Drawing for the job (mm, zero at the part's lowest x, y, z). A direction names the side the tool comes from. Coordinates: 2 decimals unless noted, no trailing zeros. Order: outer loops, then holes, each group sorted by start corner. A loop starts at its lowest first (then second) coordinate and runs counter-clockwise, first axis right, second up. Notation, with made-up numbers: M 81.25,-33.75 L 117.25,-33.75 A29 cw 117.25,-13.75 Z; hole C 7.25,-16 d7. An arc over 180 degrees is marked long. Write item = value, one per line. Start each with the question number.
Q1. Pull direction Z, two halves, no side cores. Call the marked faces 1, 2 and 3: released by +Z, released by -Z, zero draft, split by the parting line, or undercut.
Q2. 3-axis set-ups, long thin cutter, end or side, ignore diameter. For the marked faces 4 and 5: which of +Z, -Z, +X, -X, +Y, -Y reach the whole face in a straight line?
Q3. Band-saw the part on C-C on x = 7.5. Write the cut outline in (y, z).
Q4. Band-saw the part on B-B on x = 32. Write the cut outline in (y, z).
Q5. Drill centre lines: probe 1 along Z at (x, y) = (3, 13.5) (1 decimal); probe 2 along Z at (x, y) = (23.5, 14.5) (1 decimal); probe 3 along Z at (x, y) = (19.5, 15.75). Where is each one in solid material? Low to high.
Q6. Band-saw the part on A-A on x = 3.5. Write the cut outline in (y, z) (1 decimal).
Q7. Pin check, flat tips, straight feed: P1, Ø6, axis at y = 24.5, z = 15.5, coming from the +X side (1 decimal); P2, Ø3, axis at x = 3, z = 13, coming from the -Y side; P3, Ø4, axis at x = 25.5, z = 9, coming from the +Y side. Stop position of each tip, or through.
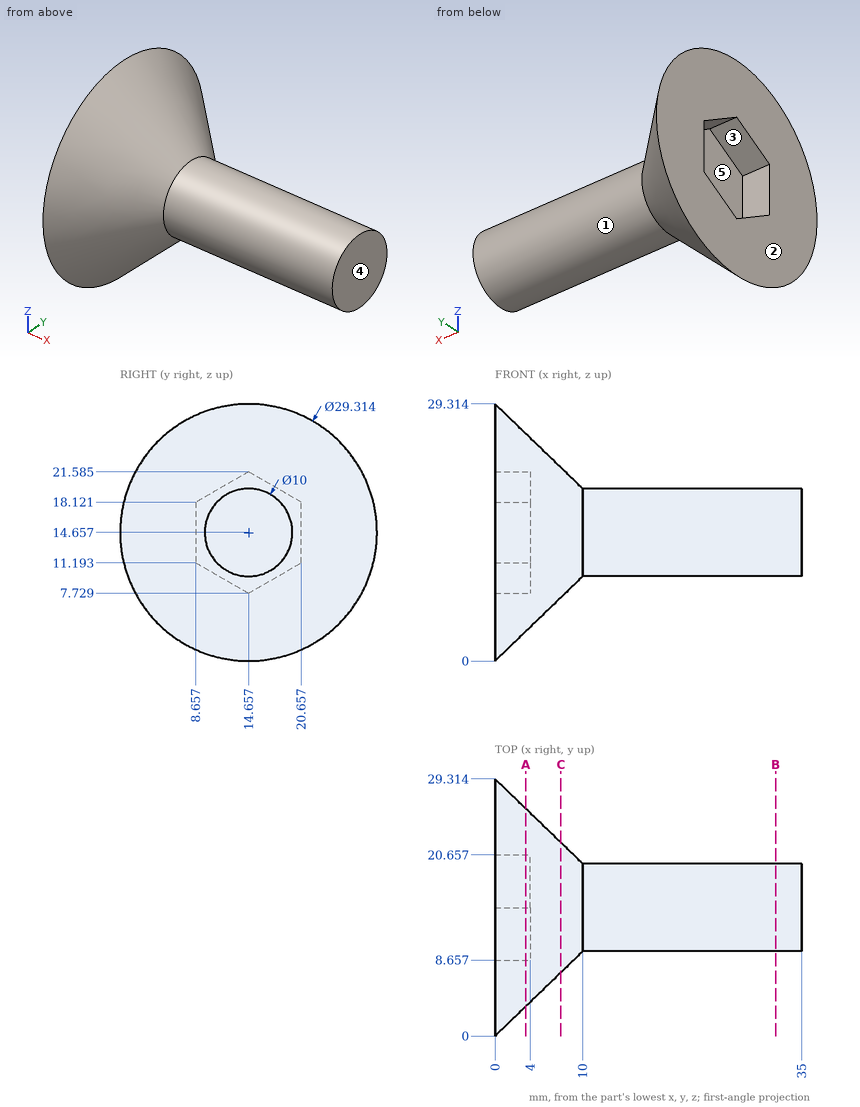
Recorded:
q1.face_1 = split by the parting line
q1.face_2 = zero draft
q1.face_3 = undercut
q2.face_4 = +Z, -Z, +X, +Y, -Y
q2.face_5 = -X
q3.outline = C 14.66,14.66 d14.83
q4.outline = C 14.66,14.66 d10
q5.probe_1 = 3 to 8.4, 20.9 to 26.4
q5.probe_2 = 9.7 to 19.7
q5.probe_3 = 9.78 to 19.54
q6.outline = C 14.7,14.7 d22.6; hole M 8.7,11.2 L 14.7,7.7 L 20.7,11.2 L 20.7,18.1 L 14.7,21.6 L 8.7,18.1 Z
q7.P1 = 8.1
q7.P2 = 1.54
q7.P3 = 18.07
